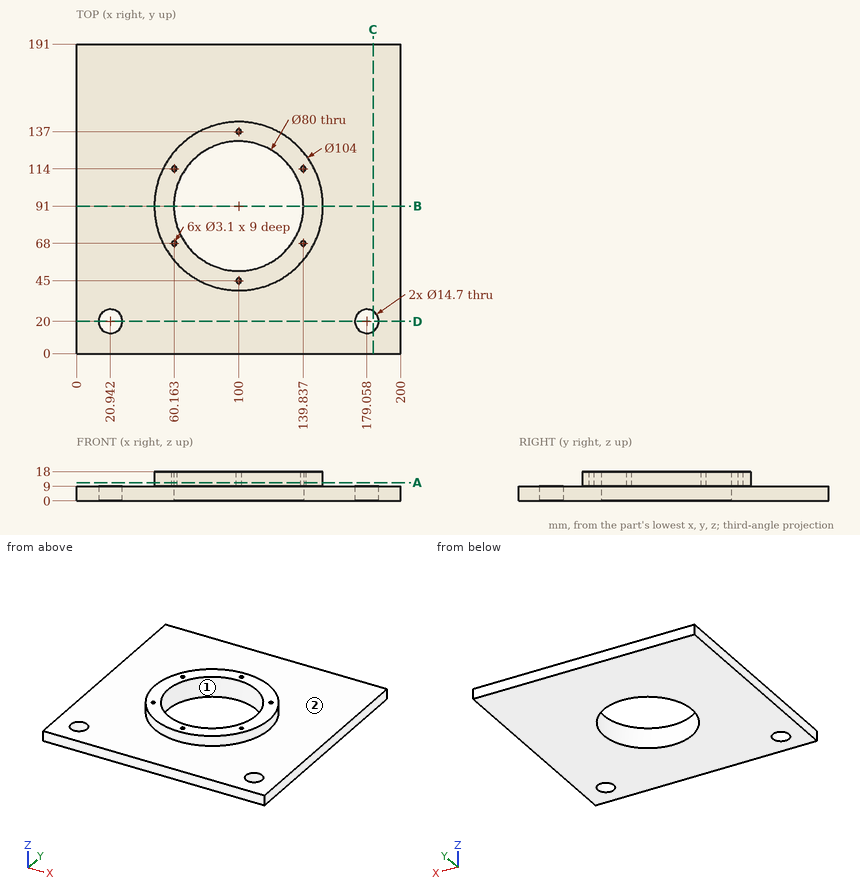
Geometry: see drawing. Coordinates: mm, zero at the bounding-box minimum. Coordinates: 2 decimals unless noted, no trailing zeros. Write each loop counter-clockwise with the first axis right and the second up, starting at its lowest first coordinate (ties: lowest second). Pieces come first, ordered by that corner, then holes.
1) Mould query, pull axis X, two halves, no side actions, for the marked faces 1 and 2. Classes: pulls with the +X half, pulls with the -X half, needs draft (parallel to the pull), parting line crosses it, or undercut.
2) Pin query (flat end, axial travel): pin 1 Ø1.9 at (x, y) = (139.84, 114) entering from +Z. Return the tip coordinate at first contact, or that it passes through.
3) Section B-B on y = 91. Output: boundary loops of the cut face in (x, z), and give its area (3 significant figures).
4) Section C-C on x = 183. Output: boundary loops of the cut face in (y, z), and give its area (3 significant figures).
5) Section A-A on z = 11.25. Output: boundary loops of the cut face in (x, y), and give its area (3 significant figures).
6) Section D-D on y = 20. Output: boundary loops of the cut face in (x, z).
7) Material intervals for line 1 along X through (y, z) = (68, 12.75) (1 decimal); line 2 along Z through (x, y) = (137, 151); line 3 along X through (y, z) = (58, 1.5) (1 decimal), sorted ascending.
Check result:
1. face 1: undercut
1. face 2: needs draft
2. pin 1: stops at z = 9
3. outline: (0, 0) - (60, 0) - (60, 18) - (48, 18) - (48, 9) - (0, 9) - close; (140, 0) - (200, 0) - (200, 9) - (152, 9) - (152, 18) - (140, 18) - close
3. area: 1,300 mm2
4. outline: (0, 0) - (13.8, 0) - (13.8, 9) - (0, 9) - close; (26.2, 0) - (191, 0) - (191, 9) - (26.2, 9) - close
4. area: 1,610 mm2
5. outline: circle Ø104 at (100, 91); hole circle Ø3.1 at (60.16, 68); hole circle Ø3.1 at (60.16, 114); hole circle Ø80 at (100, 91); hole circle Ø3.1 at (100, 45); hole circle Ø3.1 at (100, 137); hole circle Ø3.1 at (139.84, 68); hole circle Ø3.1 at (139.84, 114)
5. area: 3,420 mm2
6. outline: (0, 0) - (13.59, 0) - (13.59, 9) - (0, 9) - close; (28.29, 0) - (171.71, 0) - (171.71, 9) - (28.29, 9) - close; (186.41, 0) - (200, 0) - (200, 9) - (186.41, 9) - close
7. line 1: x = 53.4 to 58.6, 61.7 to 67.3, 132.7 to 138.3, 141.4 to 146.6
7. line 2: z = 0 to 9
7. line 3: x = 0 to 77.4, 122.6 to 200
